from build123d import *


with BuildPart() as part:
    # Sketch2 → Revolve1 (revolve)
    with BuildSketch(Plane.XY):
        with BuildLine():
            Line((44.45, 0), (49.2125, 0))
            ThreePointArc((49.2125, 0), (51.45756403, 0.92993597), (52.3875, 3.175))
            Line((52.3875, 3.175), (52.3875, 25.4))
            Line((52.3875, 25.4), (57.15, 25.4))
            Line((57.15, 25.4), (57.15, 50.8))
            ThreePointArc((57.15, 50.8), (40.411152545, 91.211152545), (0, 107.95))
            Line((0, 107.95), (0, 95.25))
            ThreePointArc((0, 95.25), (31.430896424, 82.230896424), (44.45, 50.8))
            Line((44.45, 50.8), (44.45, 0))
        make_face()
    revolve(axis=Axis((0, 107.95, 0), (0, -1, 0)))


solid = part.part
Here's how the part is built. I have some questions about the finished solid (model axes, mm). A direction names the side the tool comes from. Coordinates: 2 decimals unless noted, no trailing zeros. Loops run counter-clockwise (first coordinate to the right, second up) from the corner with the lowest first, then second, coordinate; pieces in that order, holes last.
1. Imagine slicing it at C-C, the plane y = 93.5. Please give me the cut outline in (x, z), and give its area (3 significant figures).
2. I need wall thicknesses on L1, parallel to Z at x = 0, y = 15; L2, parallel to Z at x = 0, y = 32; L3, parallel to X at y = 73, z = 34. Which ranges of each line are inside material? Lowest first, please.
3. If we mould it in two halves opening along X, with no side actions, what happens to faces 1 (the flat face through (-25.1, 25.4, -46.3)), 2 (the cylindrical face through (42.397, 25.044, 13.352)), 3 (the cylindrical face through (-57.095, 38.278, 2.513))? For each: pulls with the +X half, pulls with the -X half, needs draft (parallel to the pull), parting line crosses it, or undercut.
4. For P1, Ø5, axis at y = 96, z = -8, coming from the +X side; P2, Ø8, axis at x = -33.5, y = 84.5, coming from the +Z side; P3, Ø2, axis at x = -20, y = 78, coming from the -Z side, each with a flat end and sliding along its axis, tell me the tip position at first contact or that it passes through.
5. For faces 4 (the cylindrical face through (-11.36, 14.44, -51.14)), 5 (the flat face through (37, 0, -25)), which set-ups out of +Z, -Z, +X, -X, +Y, -Y let a thin tool reach every point of the face, with its end or its side?
Taken from the geometry:
1. outline: circle Ø75.97 at (0, 0); hole circle Ø24.7 at (0, 0)
1. area: 4,050 mm2
2. L1: z = -52.39 to -44.45, 44.45 to 52.39
2. L2: z = -57.15 to -44.45, 44.45 to 57.15
2. L3: x = -40.22 to -18.08, 18.08 to 40.22
3. face 1: needs draft
3. face 2: undercut
3. face 3: parting line crosses it
4. P1: stops at x = 37.18
4. P2: stops at z = 37.04
4. P3: stops at z = -46.83
5. face 4: -Y
5. face 5: +Z, -Z, +X, -X, -Y
